Verification items for the finished model (mm, model axes). A direction names the side the tool comes from. Round coordinates to 2 decimals unless told otherwise and drop trailing zeros. Order: outer loops, then holes, each group sorted by start corner. A loop starts at its lowest first (then second) coordinate and runs counter-clockwise, first axis right, second up. Notation, with made-up numbers: (81.25, 0.5) -> (140.25, 0.5) arc R9 cw to (140.25, 14.5) -> close; hole circle Ø11 at (53, 73.25). An arc over 180 degrees is marked (long way). Put each result on its own line as item: value.
```python
from build123d import *

# Parameters (mm, degrees)
SKETCH1_W           = 88.9
SKETCH1_H           = 88.9
BOSS_EXTRUDE1_DEPTH = 6.35
CUT_EXTRUDE3_DEPTH  = 126.88384527
SKETCH4_W           = 18.288
SKETCH4_H           = 5.588
SKETCH4_W_2         = 5.588
SKETCH4_H_2         = 18.288
CUT_EXTRUDE2_DEPTH  = 126.88384527
SKETCH7_W           = 6.731
SKETCH7_H           = 6.731
CUT_EXTRUDE4_DEPTH  = 126.88384527
FILLET1_R           = 3.81
CUT_EXTRUDE5_DEPTH  = 126.88384527


with BuildPart() as part:
    # Sketch1 → Boss-Extrude1 (new body)
    with BuildSketch(Plane(origin=(0, 0, 0), x_dir=(1, 0, 0), z_dir=(0, 1, 0))):
        with Locations((44.45, 44.45)):
            Rectangle(SKETCH1_W, SKETCH1_H)
    extrude(amount=BOSS_EXTRUDE1_DEPTH)

    # Sketch5 → Cut-Extrude3 (cut, through all)
    with BuildSketch(Plane(origin=(0, 6.35, 0), x_dir=(1, 0, 0), z_dir=(0, 1, 0))):
        Polygon((41.656, 47.244), (41.656, 53.975), (47.244, 53.975), (47.244, 47.244), (53.975, 47.244), (53.975, 41.656), (47.244, 41.656), (47.244, 34.925), (41.656, 34.925), (41.656, 41.656), (34.925, 41.656), (34.925, 47.244), align=None)
    extrude(amount=-CUT_EXTRUDE3_DEPTH, mode=Mode.SUBTRACT)

    # Sketch4 → Cut-Extrude2 (cut, through all)
    with BuildSketch(Plane(origin=(0, 6.35, 0), x_dir=(1, 0, 0), z_dir=(0, 1, 0))):
        with Locations((44.45, 86.106)):
            Rectangle(SKETCH4_W, SKETCH4_H)
        with Locations((86.106, 44.45)):
            Rectangle(SKETCH4_W_2, SKETCH4_H_2)
        with Locations((44.45, 2.794)):
            Rectangle(SKETCH4_W, SKETCH4_H)
        with Locations((2.794, 44.45)):
            Rectangle(SKETCH4_W_2, SKETCH4_H_2)
    extrude(amount=-CUT_EXTRUDE2_DEPTH, mode=Mode.SUBTRACT)

    # Sketch7 → Cut-Extrude4 (cut, through all)
    with BuildSketch(Plane(origin=(0, 6.35, 0), x_dir=(1, 0, 0), z_dir=(0, 1, 0))):
        with Locations((50.6095, 50.6095)):
            Rectangle(SKETCH7_W, SKETCH7_H)
    extrude(amount=-CUT_EXTRUDE4_DEPTH, mode=Mode.SUBTRACT)

    # Fillet1
    fillet1_edges = [part.edges().sort_by_distance(p)[0] for p in [
        (53.975, 3.175, -53.975),
    ]]
    fillet(fillet1_edges, radius=FILLET1_R)

    # Sketch8 → Cut-Extrude5 (cut, through all)
    with BuildSketch(Plane(origin=(0, 6.35, 0), x_dir=(1, 0, 0), z_dir=(0, 1, 0))):
        Polygon((5.588, 42.8625), (8.763, 42.8625), (8.763, 40.64), (11.938, 40.64), (11.938, 42.8625), (15.113, 42.8625), (15.113, 46.0375), (11.938, 46.0375), (11.938, 48.26), (8.763, 48.26), (8.763, 46.0375), (5.588, 46.0375), align=None)
        Polygon((42.8625, 83.312), (42.8625, 80.137), (40.64, 80.137), (40.64, 76.962), (42.8625, 76.962), (42.8625, 73.787), (46.0375, 73.787), (46.0375, 76.962), (48.26, 76.962), (48.26, 80.137), (46.0375, 80.137), (46.0375, 83.312), align=None)
        Polygon((83.312, 46.0375), (80.137, 46.0375), (80.137, 48.26), (76.962, 48.26), (76.962, 46.0375), (73.787, 46.0375), (73.787, 42.8625), (76.962, 42.8625), (76.962, 40.64), (80.137, 40.64), (80.137, 42.8625), (83.312, 42.8625), align=None)
        Polygon((46.0375, 5.588), (46.0375, 8.763), (48.26, 8.763), (48.26, 11.938), (46.0375, 11.938), (46.0375, 15.113), (42.8625, 15.113), (42.8625, 11.938), (40.64, 11.938), (40.64, 8.763), (42.8625, 8.763), (42.8625, 5.588), align=None)
    extrude(amount=-CUT_EXTRUDE5_DEPTH, mode=Mode.SUBTRACT)


solid = part.part
```
Item 1: Release check for a two-part mould opening along Z. For faces 5 (the face through (46.038, 3, -75)), 6 (the face through (10, 3, -48.26)), 7 (the face through (50, 3, -83.312)) record: pulls with the +Z half, pulls with the -Z half, needs draft (parallel to the pull), parting line crosses it, or undercut.
Geometry check:
face 5: needs draft
face 6: undercut
face 7: pulls with the -Z half
Item 2: Sectioned sample at A-A, the plane x = 36.5. Record the boundary of the cut face in (y, z).
Geometry check:
outline: (0, -83.31) -> (6.35, -83.31) -> (6.35, -47.24) -> (0, -47.24) -> close; (0, -41.66) -> (6.35, -41.66) -> (6.35, -5.59) -> (0, -5.59) -> close
Item 3: Depth check by flat-ended pin: pin 1 Ø1.8 at (y, z) = (3.5, -47.5) entering from +X; pin 2 Ø2 at (x, y) = (40.5, 1.5) entering from +Z; pin 3 Ø2.5 at (x, y) = (47, 3) entering from -Z. Enter the tip coordinate at first touch or a pass-through.
Geometry check:
pin 1: x = 83.31
pin 2: z = -5.59
pin 3: z = -83.31
Item 4: Sectioned sample at B-B, the plane z = -52. Record the boundary of the cut face in (x, y), then the cut area to 3 significant figures.
Geometry check:
outline: (5.59, 0) -> (41.66, 0) -> (41.66, 6.35) -> (5.59, 6.35) -> close; (53.5, 0) -> (83.31, 0) -> (83.31, 6.35) -> (53.5, 6.35) -> close
area: 418 mm2
Item 5: Material ranges on line 1 along X through (y, z) = (4, -41.5); line 2 along X through (y, z) = (6.25, -85); line 3 along X through (y, z) = (1, -40), recorded low to high.
Geometry check:
line 1: 5.59 to 8.76, 11.94 to 41.66, 47.24 to 76.96, 80.14 to 83.31
line 2: 0 to 35.31, 53.59 to 88.9
line 3: 5.59 to 41.66, 47.24 to 83.31
Item 6: Tool access check on faces 1 (the face through (46, 3, -53.975)), 2 (the face through (83.312, 3, -39)), 3 (the face through (53.594, 3, -3)), 4 (the face through (14, 3, -46.038)). Record the directions out of +Z, -Z, +X, -X, +Y, -Y that give a thin tool (end or side, any length) a straight path to the whole face; none if there is none.
Geometry check:
face 1: +Y, -Y
face 2: +X, +Y, -Y
face 3: +Z, +Y, -Y
face 4: -X, +Y, -Y
